The listing builds one solid part. Answer for the finished solid, in the listing's coordinates (mm). Face numbers are marked on the shaded views. A direction names the side the tool comes from. Give positions to 0.01 mm unless a question says otherwise; leave off trailing zeros. Order: outer loops, then holes, each group sorted by start corner. A loop starts at its lowest first (then second) coordinate and runs counter-clockwise, first axis right, second up. Notation, with made-up numbers: (-40, -39) - (-18, -39) arc R28 cw to (-18, -13) - close; hole circle Ø8 at (-15, 32.25). An arc over 180 degrees is marked (long way). Answer as CSV lines item,"result". Start each with the question number.
1. Section B-B on z = 0 is taken. Give the vertices of the cut face in (x, y), and give its area (3 significant figures).
2. Which of the six approach directions +Z, -Z, +X, -X, +Y, -Y give full straight-line access (tool end or side, diameter ignored) to the marked faces 4, 5 and 6?
3. Flat-ended cylindrical pins translate along their axes: pin 1 (0.6 mm diameter, centred on x = 12, y = 1.5, fed in from +Z); pin 2 (12 mm diameter, centred on x = 16.5, z = 16.5, fed in from +Y); pin 3 (9.5 mm diameter, centred on x = 0, z = -18.86, fed in from +Y); pin 4 (1 mm diameter, centred on x = -12.5, y = 1.5, fed in from -Z). Find the tip coordinate at first contact, or state that the pin passes through.
4. Section D-D on y = 5 is taken. Give the vertices of the cut face in (x, z), and give its area (3 significant figures).
5. Consider line 1 along X through (y, z) = (0.55, 0); line 2 along Z through (x, y) = (2.5, 3); line 3 along Z through (x, y) = (-2, 4.75). Determine where each line is inside the solid, lowest interval first. Write a range as [from, to].
6. Determine the mould class of the marked faces 1, 2 and 3 for opening direction Z: +Z half, -Z half, draft (parallel to the pull), parting line (faces both ways), or undercut.
7. Section A-A on x = 0 is taken. Give the vertices of the cut face in (y, z).
8. Section C-C on x = -18 is taken. Give the vertices of the cut face in (y, z), and give its area (3 significant figures).
from build123d import *

# Parameters (mm, degrees)
SKETCH1_W           = 17
SKETCH1_H           = 55
SKETCH1_R           = 7.55
SKETCH1_W_2         = 14
SKETCH1_H_2         = 9
SKETCH1_R_2         = 1.5
BOSS_EXTRUDE1_DEPTH = 2
BOSS_EXTRUDE2_START = 2
SKETCH1_4_W         = 17
SKETCH1_4_H         = 55
SKETCH1_4_R         = 7.55
BOSS_EXTRUDE2_DEPTH = 1.94
BOSS_EXTRUDE3_START = 3.94
SKETCH1_5_W         = 17
SKETCH1_5_H         = 55
SKETCH1_5_R         = 7.55
BOSS_EXTRUDE3_DEPTH = 2.25
SKETCH3_R           = 3
CUT_EXTRUDE1_DEPTH  = 37.06682825


with BuildPart() as part:
    # Sketch1 → Boss-Extrude1 (new body)
    # profile 1 of 5: a face of its own
    with BuildSketch(Plane(origin=(0, 0, 0), x_dir=(1, 0, 0), z_dir=(0, 1, 0))):
        Rectangle(SKETCH1_W, SKETCH1_H)
        with Locations((0, -18.8625)):
            Circle(SKETCH1_R, mode=Mode.SUBTRACT)
        with Locations((0, 18.8625)):
            Circle(SKETCH1_R, mode=Mode.SUBTRACT)
    # profile 2 of 5: a face of its own
    with BuildSketch(Plane(origin=(0, 0, 0), x_dir=(1, 0, 0), z_dir=(0, 1, 0))):
        with Locations((15.5, 0)):
            Rectangle(SKETCH1_W_2, SKETCH1_H_2)
        with Locations(Location((18, 0, 0), (0, 0, 270))):
            Circle(SKETCH1_R_2, mode=Mode.SUBTRACT)
    # profile 3 of 5: a face of its own
    with BuildSketch(Plane(origin=(0, 0, 0), x_dir=(1, 0, 0), z_dir=(0, 1, 0))):
        with Locations((-15.5, 0)):
            Rectangle(SKETCH1_W_2, SKETCH1_H_2)
        with Locations(Location((-18, 0, 0), (0, 0, 270))):
            Circle(SKETCH1_R_2, mode=Mode.SUBTRACT)
    # profile 4 of 5: a face of its own
    with BuildSketch(Plane(origin=(0, 0, 0), x_dir=(1, 0, 0), z_dir=(0, 1, 0))):
        with Locations((0, -18.8625)):
            Circle(SKETCH1_R)
    # profile 5 of 5: a face of its own
    with BuildSketch(Plane(origin=(0, 0, 0), x_dir=(1, 0, 0), z_dir=(0, 1, 0))):
        with Locations((0, 18.8625)):
            Circle(SKETCH1_R)
    extrude(amount=BOSS_EXTRUDE1_DEPTH)

    # Sketch1<4> → Boss-Extrude2 (add)
    # profile 1 of 3: a face of its own
    with BuildSketch(Plane(origin=(0, 0, 0), x_dir=(1, 0, 0), z_dir=(0, 1, 0)).offset(BOSS_EXTRUDE2_START)):
        Rectangle(SKETCH1_4_W, SKETCH1_4_H)
        with Locations((0, -18.8625)):
            Circle(SKETCH1_4_R, mode=Mode.SUBTRACT)
        with Locations((0, 18.8625)):
            Circle(SKETCH1_4_R, mode=Mode.SUBTRACT)
    # profile 2 of 3: a face of its own
    with BuildSketch(Plane(origin=(0, 0, 0), x_dir=(1, 0, 0), z_dir=(0, 1, 0)).offset(BOSS_EXTRUDE2_START)):
        with Locations((0, -18.8625)):
            Circle(SKETCH1_4_R)
    # profile 3 of 3: a face of its own
    with BuildSketch(Plane(origin=(0, 0, 0), x_dir=(1, 0, 0), z_dir=(0, 1, 0)).offset(BOSS_EXTRUDE2_START)):
        with Locations((0, 18.8625)):
            Circle(SKETCH1_4_R)
    extrude(amount=BOSS_EXTRUDE2_DEPTH)

    # Sketch1<5> → Boss-Extrude3 (add)
    with BuildSketch(Plane(origin=(0, 0, 0), x_dir=(1, 0, 0), z_dir=(0, 1, 0)).offset(BOSS_EXTRUDE3_START)):
        Rectangle(SKETCH1_5_W, SKETCH1_5_H)
        with Locations(Location((0, -18.8625, 0), (0, 0, 90))):
            Circle(SKETCH1_5_R, mode=Mode.SUBTRACT)
        with Locations(Location((0, 18.8625, 0), (0, 0, 90))):
            Circle(SKETCH1_5_R, mode=Mode.SUBTRACT)
    extrude(amount=BOSS_EXTRUDE3_DEPTH)

    # Sketch3 → Cut-Extrude1 (cut, through all)
    with BuildSketch(Plane.XZ):
        with Locations(Location((0, -18.8625, 0), (0, 0, 270))):
            Circle(SKETCH3_R)
        with Locations(Location((0, 18.8625, 0), (0, 0, 270))):
            Circle(SKETCH3_R)
    extrude(amount=-CUT_EXTRUDE1_DEPTH, mode=Mode.SUBTRACT)


solid = part.part
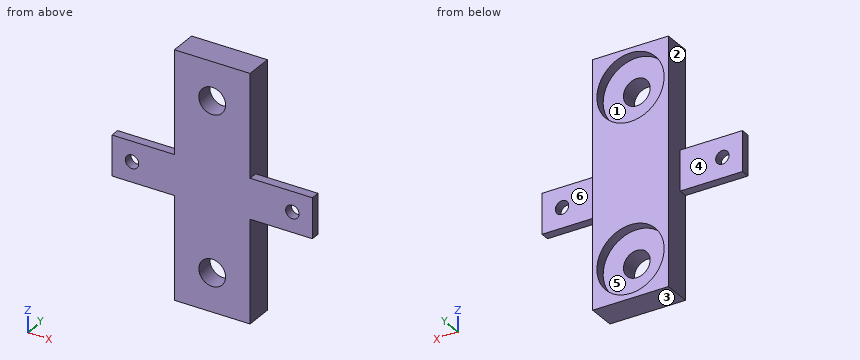
Checks:
1,outline,"(-22.5, 0) - (-19.5, 0) - (-19.5, 2) - (-22.5, 2) - close; (-16.5, 0) - (16.5, 0) - (16.5, 2) - (8.5, 2) - (8.5, 6.19) - (-8.5, 6.19) - (-8.5, 2) - (-16.5, 2) - close; (19.5, 0) - (22.5, 0) - (22.5, 2) - (19.5, 2) - close"
1,area,"149 mm²"
2,face 4,"+Z, -Z, -X, +Y"
2,face 5,"+Y"
2,face 6,"+Z, -Z, +X, +Y"
3,pin 1,"stops at z = 4.5"
3,pin 2,"passes through"
3,pin 3,"stops at y = 3.94"
3,pin 4,"stops at z = -4.5"
4,outline,"(-8.5, -27.5) - (8.5, -27.5) - (8.5, 27.5) - (-8.5, 27.5) - close; hole circle Ø15.1 at (0, -18.86); hole circle Ø15.1 at (0, 18.86)"
4,area,"577 mm²"
5,line 1,"x = [-22.5, -19.5], [-16.5, 16.5], [19.5, 22.5]"
5,line 2,"z = [-27.5, -20.52], [-17.2, 17.2], [20.52, 27.5]"
5,line 3,"z = [-27.5, -26.14], [-11.58, 11.58], [26.14, 27.5]"
6,face 1,"undercut"
6,face 2,"draft"
6,face 3,"-Z half"
7,outline,"(0, -27.5) - (6.19, -27.5) - (6.19, -26.41) - (3.94, -26.41) - (3.94, -21.86) - (0, -21.86) - close; (0, -15.86) - (3.94, -15.86) - (3.94, -11.31) - (6.19, -11.31) - (6.19, 11.31) - (3.94, 11.31) - (3.94, 15.86) - (0, 15.86) - close; (0, 21.86) - (3.94, 21.86) - (3.94, 26.41) - (6.19, 26.41) - (6.19, 27.5) - (0, 27.5) - close"
8,outline,"(0, -4.5) - (2, -4.5) - (2, -1.5) - (0, -1.5) - close; (0, 1.5) - (2, 1.5) - (2, 4.5) - (0, 4.5) - close"
8,area,"12.0 mm²"
